Design review of the part built by this model. Coordinates are the model's own, in mm. Face numbers are marked on the shaded views. A direction names the side the tool comes from. Coordinates: 2 decimals unless noted, no trailing zeros. Write each loop counter-clockwise with the first axis right and the second up, starting at its lowest first coordinate (ties: lowest second). Pieces come first, ordered by that corner, then holes. Notation, with made-up numbers: (-27, -16) -> (31, -16) arc R17 cw to (31, -8) -> close; hole circle Ø9 at (82, 64.25). An arc over 180 degrees is marked (long way). Answer in a Markdown table with one row per item. Add a question column.
Item 1: For the marked faces 1 and 2, list the 3-axis set-ups (+Z, -Z, +X, -X, +Y, -Y) from which the entire face can be reached by the end or side of a thin tool; tool diameter is ignored.
Item 2: Clearance check with flat-ended pins moving along their axes: P1, Ø3.5, axis at y = 10, z = 9, coming from the -X side; P2, Ø1, axis at x = 17, z = 11, coming from the +Y side; P3, Ø3, axis at y = 9.5, z = 2, coming from the +X side; P4, Ø1, axis at x = 14, y = 3.5, coming from the -Z side. State where each tip first meets the part, or that it passes through.
Item 3: Take a section at D-D, the plane z = 4.75. Write out the cut boundary in (x, y).
Item 4: Take a section at A-A, the plane x = 10. Write out the cut boundary in (y, z).
Item 5: To check wall thickness, follow line 1 (Z direction, x = 10, y = 0.8); line 2 (X direction, y = 15.25, z = 9). State the ranges of each line that lie inside material, in increasing order.
Item 6: Take a section at B-B, the plane y = 10. Write out the cut boundary in (x, z), and give its area (4 significant figures).
Item 7: Take a section at C-C, the plane z = 8.5. Write out the cut boundary in (x, y).
from build123d import *

# Parameters (mm, degrees)
EXTRUSION1_DEPTH = 17.5
ESQUISSE7_R      = 1.5
EXTRUSION7_DEPTH = 33.380549717
ESQUISSE9_R      = 1.5
EXTRUSION8_DEPTH = 33.380549717
ESQUISSE10_W     = 4
ESQUISSE10_H     = 6
EXTRUSION9_DEPTH = 6


with BuildPart() as part:
    # Esquisse1 → Extrusion1 (new body)
    with BuildSketch(Plane.XY):
        Polygon((0, 0), (20, 0), (20, 1.5), (1.5, 1.5), (1.5, 20), (0, 20), align=None)
    extrude(amount=EXTRUSION1_DEPTH)

    # Esquisse7 → Extrusion7 (cut, through all)
    with BuildSketch(Plane(origin=(0, 1.5, 0), x_dir=(-1, 0, 0), z_dir=(0, 1, 0))):
        with Locations((-10, 7.5)):
            Circle(ESQUISSE7_R)
    extrude(amount=-EXTRUSION7_DEPTH, mode=Mode.SUBTRACT)

    # Esquisse9 → Extrusion8 (cut, through all)
    with BuildSketch(Plane(origin=(1.5, 0, 0), x_dir=(0, 0, -1), z_dir=(1, 0, 0))):
        with Locations(Location((-9, 10, 0), (0, 0, 90))):
            Circle(ESQUISSE9_R)
    extrude(amount=-EXTRUSION8_DEPTH, mode=Mode.SUBTRACT)

    # Esquisse10 → Extrusion9 (cut)
    with BuildSketch(Plane.ZY):
        with Locations((2, 3)):
            Rectangle(ESQUISSE10_W, ESQUISSE10_H)
    extrude(amount=-EXTRUSION9_DEPTH, mode=Mode.SUBTRACT)


solid = part.part
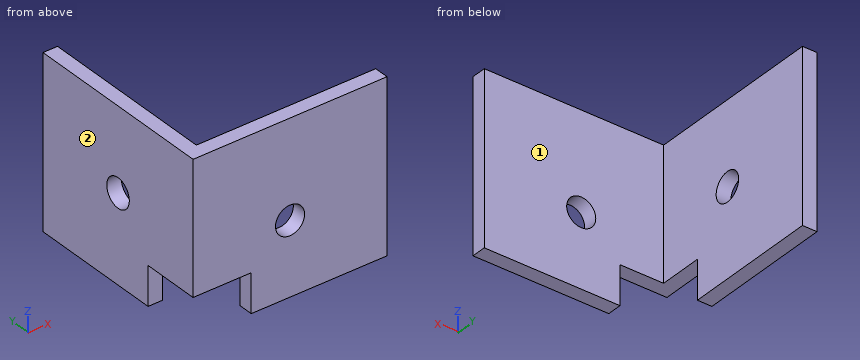
Answers:
| question | item | result |
|---|---|---|
| 1 | face 1 | +Z, -Z, +X, +Y |
| 1 | face 2 | +Z, -Z, -X, +Y, -Y |
| 2 | P1 | stops at x = 0 |
| 2 | P2 | stops at y = 1.5 |
| 2 | P3 | stops at x = 1.5 |
| 2 | P4 | passes through |
| 3 | outline | (0, 0) -> (20, 0) -> (20, 1.5) -> (1.5, 1.5) -> (1.5, 20) -> (0, 20) -> close |
| 4 | outline | (0, 0) -> (1.5, 0) -> (1.5, 6) -> (0, 6) -> close; (0, 9) -> (1.5, 9) -> (1.5, 17.5) -> (0, 17.5) -> close |
| 5 | line 1 | z = 0 to 6, 9 to 17.5 |
| 5 | line 2 | x = 0 to 1.5 |
| 6 | outline | (0, 0) -> (1.5, 0) -> (1.5, 7.5) -> (0, 7.5) -> close; (0, 10.5) -> (1.5, 10.5) -> (1.5, 17.5) -> (0, 17.5) -> close |
| 6 | area | 21.75 mm^2 |
| 7 | outline | (0, 0) -> (8.88, 0) -> (8.88, 1.5) -> (1.5, 1.5) -> (1.5, 8.59) -> (0, 8.59) -> close; (0, 11.41) -> (1.5, 11.41) -> (1.5, 20) -> (0, 20) -> close; (11.12, 0) -> (20, 0) -> (20, 1.5) -> (11.12, 1.5) -> close |
